Source: CAD feature listing. Evaluate the final solid. Frame: model axes, mm. Face numbers are marked on the shaded views. A direction names the side the tool comes from. Round coordinates to 2 decimals unless told otherwise and drop trailing zeros. Order: outer loops, then holes, each group sorted by start corner. A loop starts at its lowest first (then second) coordinate and runs counter-clockwise, first axis right, second up. Notation, with made-up numbers: (3, 38) -> (21, 38) arc R22 cw to (21, 66) -> close; hole circle Ø11 at (81.25, -27.5). An arc over 180 degrees is marked (long way). One line per item, written item: value. Start each with the question number.
1) Section D-D (y = -29.5). Return the cut outline in (x, z).
2) Reachability of the marked faces 1 and 2 from +Z, -Z, +X, -X, +Y, -Y: full face, straight path, thin tool, end or side. Return the list, or none.
3) Section A-A (x = 0). Return the cut outline in (y, z).
4) Pin query (flat end, axial travel): P1, Ø10, axis at y = -16, z = -7, coming from the +X side; P2, Ø3, axis at x = -17.32, z = -10, coming from the -Y side; P3, Ø8, axis at x = -13.5, y = -9, coming from the +Z side. Return the tip coordinate at first contact, or that it passes through.
5) Section B-B (z = 0). Return the cut outline in (x, y), and give its area (3 significant figures).
6) Section C-C (z = -10). Return the cut outline in (x, y).
7) Ray query, L1, parallel to Z at x = 0, y = 1.7; L2, parallel to Y at x = 12.5, z = 15; L3, parallel to Y at x = 0, z = -12.5. Return the intervals inside material, ascending.
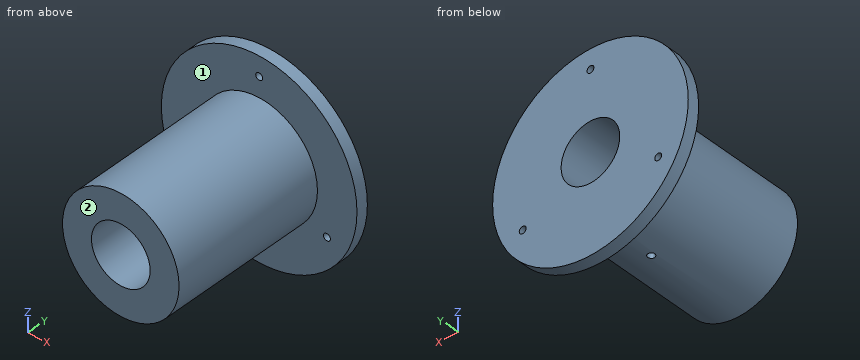
```python
from build123d import *

# Parameters (mm, degrees)
F0_R     = 14.9
F0_R_2   = 7.5
F1_DEPTH = 40
F0_R_3   = 25
F0_R_4   = 0.88
F2_DEPTH = 3
F3_R     = 0.88
F4_DEPTH = 25


with BuildPart() as f1:
    # F0 (on Front) → F1 (new body)
    with BuildSketch(Plane.XZ):
        Circle(F0_R)
        Circle(F0_R_2, mode=Mode.SUBTRACT)
    extrude(amount=F1_DEPTH)

    # F0 (on Front) → F2 (join)
    with BuildSketch(Plane.XZ):
        Circle(F0_R_3)
        with Locations((-17.320508, -10)):
            Circle(F0_R_4, mode=Mode.SUBTRACT)
        with Locations((17.320508, -10)):
            Circle(F0_R_4, mode=Mode.SUBTRACT)
        Circle(F0_R, mode=Mode.SUBTRACT)
        with Locations((0, 20)):
            Circle(F0_R_4, mode=Mode.SUBTRACT)
        Circle(F0_R)
        Circle(F0_R_2, mode=Mode.SUBTRACT)
    extrude(amount=-F2_DEPTH)

    # F3 (on Top) → F4 (cut)
    with BuildSketch(Plane.XY):
        with Locations((0, -14.562329)):
            Circle(F3_R)
    extrude(amount=-F4_DEPTH, mode=Mode.SUBTRACT)


solid = f1.part
```
Findings:
1. outline: circle Ø29.8 at (0, 0); hole circle Ø15 at (0, 0)
2. face 1: -Y
2. face 2: +Z, -Z, +X, -X, -Y
3. outline: (-40, -14.9) -> (-15.44, -14.9) -> (-15.44, -7.5) -> (-40, -7.5) -> close; (-40, 7.5) -> (3, 7.5) -> (3, 19.12) -> (0, 19.12) -> (0, 14.9) -> (-40, 14.9) -> close; (-13.68, -14.9) -> (0, -14.9) -> (0, -25) -> (3, -25) -> (3, -7.5) -> (-13.68, -7.5) -> close; (0, 20.88) -> (3, 20.88) -> (3, 25) -> (0, 25) -> close
4. P1: x = 14.77
4. P2: y = 0
4. P3: z = 11.48
5. outline: (-25, 0) -> (-14.9, 0) -> (-14.9, -40) -> (-7.5, -40) -> (-7.5, 3) -> (-25, 3) -> close; (7.5, -40) -> (14.9, -40) -> (14.9, 0) -> (25, 0) -> (25, 3) -> (7.5, 3) -> close
5. area: 697 mm2
6. outline: (-22.91, 0) -> (-18.2, 0) -> (-18.2, 3) -> (-22.91, 3) -> close; (-16.44, 0) -> (-11.05, 0) -> (-11.05, -40) -> (11.05, -40) -> (11.05, 0) -> (16.44, 0) -> (16.44, 3) -> (-16.44, 3) -> close; (18.2, 0) -> (22.91, 0) -> (22.91, 3) -> (18.2, 3) -> close; hole circle Ø1.76 at (0, -14.56)
7. L1: -25 to -7.5, 7.5 to 19.12, 20.88 to 25
7. L2: 0 to 3
7. L3: -40 to -15.44, -13.68 to 3
